Autodesk Inventor part; units mm, degrees
ref_plane "Arbeitsebene1" through (0, 10, 0) normal (0, 1, 0) x (-1, 0, 0)
ref_plane "YZ Plane" through (0, 0, 0) normal (1, 0, 0) x (0, 1, 0)
ref_plane "XZ Plane" through (0, 0, 0) normal (0, 1, 0) x (-1, 0, 0)
sketch "Skizze1" plane through (0, 0, 0) normal (0, 0, 1) x (1, 0, 0)
  line L0 (0, -20.5159) -> (0, 20.5159)
  line L1 (-23.1, 0) -> (23.1, 0)
  circle A0 centre (0, 0) radius 2.5
  arc A1 (-3, 4) -> (-3, -4) centre (0, 0) ccw
  arc A2 (7.5831, -14.6542) -> (7.5831, 14.6542) centre (0, 0) ccw
  line L2 (-3.5355, 3.5355) -> (7.5831, 14.6542)
  line L3 (-3.5355, -3.5355) -> (7.5831, -14.6542)
  line L4 (-3, 4) -> (-12.5, 4)
  line L5 (-3, -4) -> (-12.5, -4)
  arc A3 (-12.5, 4) -> (-12.5, -4) centre (-12.5, 0) ccw
  dimension "d0" = 5
  dimension "d1" = 10
  dimension "d3" = 33
  dimension "d4" = 90
  dimension "d5" = 4
  dimension "d6" = 12.5
extrude "Extrusion1" add sketch "Skizze1" along normal blind 4 contours L3 L5 A1 L1 A0 L0 | L0 A0 L1 A2 L3 | L5 A3 L1 A1 L3 | L3 A1 L5 | L1 A1 L4 L2 L0 A0 | A0 L0 L2 A2 L1 | L1 A3 L4 L2 A1 | L2 L4 A1
fillet "Rundung1" radius 2.5 2 edges at (7.5831, 14.6542, 2) (7.5831, -14.6542, 2)
sketch "Skizze2" plane through (0, 0, 4) normal (0, 0, 1) x (1, 0, 0)
  arc A0 (-12.5, 4) -> (-12.5, -4) centre (-12.5, 0) ccw
  point P0 (0, 0)
hole "Bohrung1" at (-12.5, 0, 4) direction (0, 0, -1) diameter 2.459 end through all
sketch "Skizze3" plane through (0, 0, 4) normal (0, 0, 1) x (1, 0, 0)
  line L0 (0, -19.6114) -> (0, 19.6114)
  line L1 (-23.1, 0) -> (23.1, 0)
  line L2 (-12.5, -4) -> (-3.0711, -4)
  circle A0 centre (0, 0) radius 5.043
  circle A1 centre (0, 0) radius 2.5
  dimension "d17" = 5
extrude "Extrusion2" add sketch "Skizze3" along normal blind 1 contours A0 L1 A1 L0 | L0 A1 L1 A0 | L1 A1 L0 A0 | L1 A0 L0 A1
ref_plane "Arbeitsebene1" through (0, 10, 0) normal (0, 1, 0) x (-1, 0, 0)
sketch "Skizze7" plane through (0, 10, 0) normal (0, 1, 0) x (-1, 0, 0)
  line L0 (0, -1) -> (0, 6)
  line L1 (23.1, 0) -> (-23.1, 0)
  line L2 (12.5, 0) -> (12.5, 4)
  point P0 (0, 0)
  point P1 (0, 2)
  dimension "d30" = 2
hole "Bohrung3" at (0, 10, 2) direction (0, -1, 0) diameter 3.5 depth 4.6
sketch "Skizze8" plane through (0, 5.4, 2) normal (0, 1, 0) x (1, 0, 0)
  line L0 (0, 3) -> (0, -4)
  line L1 (23.1, 2) -> (-23.1, 2)
  point P0 (0, 2)
  point P1 (0, 0)
  dimension "d38" = 2
hole "Bohrung4" at (0, 5.4, 2) direction (0, -1, 0) diameter 2.459 end up to surface
properties part number "Kurbel 20"
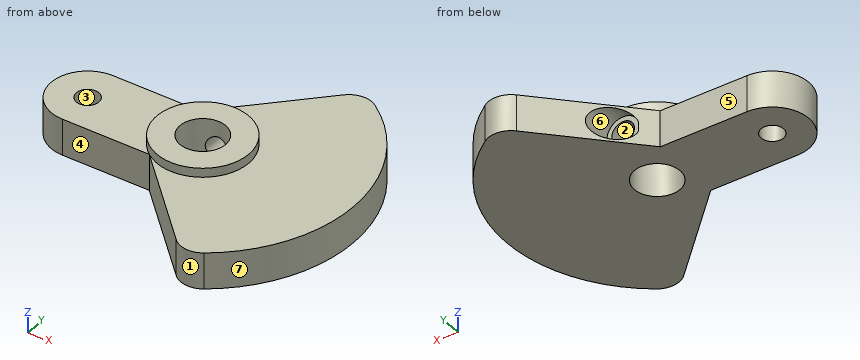
Here's how the part is built. I have some questions about the finished solid (model axes, mm). Face numbers are marked on the shaded views. A direction names the side the tool comes from. Give positions to 0.01 mm unless a question says otherwise; leave off trailing zeros. Order: outer loops, then holes, each group sorted by start corner. A loop starts at its lowest first (then second) coordinate and runs counter-clockwise, first axis right, second up. Notation, with made-up numbers: (-8, 39) -> (-3, 39) arc R6 cw to (-3, 45) -> close; hole circle Ø1 at (43, 47). An arc over 180 degrees is marked (long way). Use a Markdown table: item, result. Add a question column.
Item 1: Imagine slicing it at D-D on y = 7.75. Please give me the cut outline in (x, z), plus the area to 3 significant figures.
Item 2: Imagine slicing it at A-A on z = 2. Please give me the cut outline in (x, y).
Item 3: If we mould it in two halves opening along X, with no side actions, what happens to the marked faces 1, 2, 3 and 4? For each: pulls with the +X half, pulls with the -X half, needs draft (parallel to the pull), parting line crosses it, or undercut.
Item 4: Imagine slicing it at C-C on x = -12. Please give me the cut outline in (y, z).
Item 5: Imagine slicing it at B-B on x = 0. Please give me the cut outline in (y, z), plus the area to 3 significant figures.
Item 6: I need wall thicknesses on line 1 (X direction, y = 0, z = 3.2); line 2 (Y direction, x = -12.5, z = 2.5); line 3 (X direction, y = -0.75, z = 0.45). Which ranges of each line are inside material? Lowest first, please.
Item 7: Will these pins go through, and if not, where does the flat tip stop? pin 1 (1 mm diameter, centred on x = -3, z = 2, fed in from +Y); pin 2 (3 mm diameter, centred on x = -8, z = 2, fed in from -Y); pin 3 (4 mm diameter, centred on x = -12.5, y = 0, fed in from +Z).
Item 8: For the marked faces 5, 6 and 7, which set-ups out of +Z, -Z, +X, -X, +Y, -Y let a thin tool reach every point of the face, with its end or its side?
Data:
| question | item | result |
|---|---|---|
| 1 | outline | (0.68, 0) -> (14.57, 0) -> (14.57, 4) -> (0.68, 4) -> (0.68, 3.61) arc R1.75 cw to (0.68, 0.39) -> close |
| 1 | area | 53.1 mm² |
| 2 | outline | (-12.5, -4) -> (-3.07, -4) -> (6.2, -13.28) arc R2.5 ccw to (9.4, -13.56) arc R16.5 ccw to (9.4, 13.56) arc R2.5 ccw to (6.2, 13.28) -> (1.75, 8.82) -> (1.75, 5.4) -> (1.23, 5.4) -> (1.23, 2.18) arc R2.5 cw (long way) to (-1.23, 2.18) -> (-1.23, 5.4) -> (-1.67, 5.4) -> (-3.07, 4) -> (-12.5, 4) arc R4 ccw to start; hole circle Ø2.46 at (-12.5, 0) |
| 3 | face 1 | parting line crosses it |
| 3 | face 2 | undercut |
| 3 | face 3 | undercut |
| 3 | face 4 | needs draft |
| 4 | outline | (-4, 0) -> (-1.12, 0) -> (-1.12, 4) -> (-4, 4) -> close; (1.12, 0) -> (4, 0) -> (4, 4) -> (1.12, 4) -> close |
| 5 | outline | (-7.07, 0) -> (-2.5, 0) -> (-2.5, 5) -> (-5.04, 5) -> (-5.04, 4) -> (-7.07, 4) -> close; (2.5, 0) -> (7.07, 0) -> (7.07, 0.25) -> (5.4, 0.25) -> (5.4, 0.77) -> (2.5, 0.77) -> close; (2.5, 3.23) -> (5.4, 3.23) -> (5.4, 3.75) -> (7.07, 3.75) -> (7.07, 4) -> (5.04, 4) -> (5.04, 5) -> (2.5, 5) -> close |
| 5 | area | 28.7 mm² |
| 6 | line 1 | x = -16.5 to -13.73, -11.27 to -2.5, 2.5 to 16.5 |
| 6 | line 2 | y = -4 to -1.23, 1.23 to 4 |
| 6 | line 3 | x = -16.43 to -13.47, -11.53 to -2.38, 2.38 to 16.48 |
| 7 | pin 1 | stops at y = 4.57 |
| 7 | pin 2 | stops at y = -4 |
| 7 | pin 3 | stops at z = 4 |
| 8 | face 5 | +Z, -Z, -X, +Y |
| 8 | face 6 | +Y |
| 8 | face 7 | +Z, -Z, +X |
